```python
from build123d import *

# Parameters (mm, degrees)
SKETCH1_R           = 4
SKETCH1_R_2         = 1.5
SKETCH1_R_3         = 2
BOSS_EXTRUDE1_DEPTH = 2.5
SKETCH2_R           = 2.1
BOSS_EXTRUDE2_DEPTH = 9.5


with BuildPart() as part:
    # Sketch1 → Boss-Extrude1 (new body)
    with BuildSketch(Plane.XY):
        with BuildLine():
            Line((-24, 5.07179677), (-24, 21.07179677))
            Line((-24, 21.07179677), (-4, 33.07179677))
            Line((-4, 33.07179677), (4, 33.07179677))
            Line((4, 33.07179677), (24, 21.07179677))
            Line((24, 21.07179677), (24, 5.07179677))
            Line((24, 5.07179677), (8, -6.92820323))
            Line((8, -6.92820323), (8, -34.92820323))
            ThreePointArc((8, -34.92820323), (7.414213562, -36.342416793), (6, -36.92820323))
            Line((6, -36.92820323), (-6, -36.92820323))
            ThreePointArc((-6, -36.92820323), (-7.414213562, -36.342416793), (-8, -34.92820323))
            Line((-8, -34.92820323), (-8, -6.92820323))
            Line((-8, -6.92820323), (-24, 5.07179677))
        make_face()
        with Locations((-12, 14.07179677)):
            Circle(SKETCH1_R, mode=Mode.SUBTRACT)
        with Locations((-4, 14.07179677)):
            Circle(SKETCH1_R_2, mode=Mode.SUBTRACT)
        with Locations((4, 14.07179677)):
            Circle(SKETCH1_R_2, mode=Mode.SUBTRACT)
        with Locations((0, 29.07179677)):
            Circle(SKETCH1_R_2, mode=Mode.SUBTRACT)
        with Locations((20, 17.07179677)):
            Circle(SKETCH1_R_2, mode=Mode.SUBTRACT)
        with Locations((20, 9.07179677)):
            Circle(SKETCH1_R_2, mode=Mode.SUBTRACT)
        with Locations((-20, 17.07179677)):
            Circle(SKETCH1_R_2, mode=Mode.SUBTRACT)
        with Locations((-20, 9.07179677)):
            Circle(SKETCH1_R_2, mode=Mode.SUBTRACT)
        with Locations((13, 14.07179677)):
            Circle(SKETCH1_R_3, mode=Mode.SUBTRACT)
        with BuildLine():
            Line((4, -30.92820323), (-4, -30.92820323))
            Line((-4, -30.92820323), (-4, -6.92820323))
            ThreePointArc((-4, -6.92820323), (0, 8), (4, -6.92820323))
            Line((4, -6.92820323), (4, -30.92820323))
        make_face(mode=Mode.SUBTRACT)
        with BuildLine():
            Line((-5, 25.07179677), (5, 25.07179677))
            ThreePointArc((5, 25.07179677), (6.414213562, 24.486010332), (7, 23.07179677))
            Line((7, 23.07179677), (7, 20.07179677))
            ThreePointArc((7, 20.07179677), (6.414213562, 18.657583207), (5, 18.07179677))
            Line((5, 18.07179677), (-5, 18.07179677))
            ThreePointArc((-5, 18.07179677), (-6.414213562, 18.657583207), (-7, 20.07179677))
            Line((-7, 20.07179677), (-7, 23.07179677))
            ThreePointArc((-7, 23.07179677), (-6.414213562, 24.486010332), (-5, 25.07179677))
        make_face(mode=Mode.SUBTRACT)
    extrude(amount=BOSS_EXTRUDE1_DEPTH)

    # Sketch2 → Boss-Extrude2 (add)
    with BuildSketch(Plane(origin=(0, 0, 0), x_dir=(-1, 0, 0), z_dir=(0, 0, -1))):
        with Locations(Location((-5, -32.16164975, 0), (0, 0, 61.563109851))):
            Circle(SKETCH2_R)
        with Locations(Location((5, -32.16164975, 0), (0, 0, 144.030430851))):
            Circle(SKETCH2_R)
    extrude(amount=BOSS_EXTRUDE2_DEPTH)


solid = part.part
```
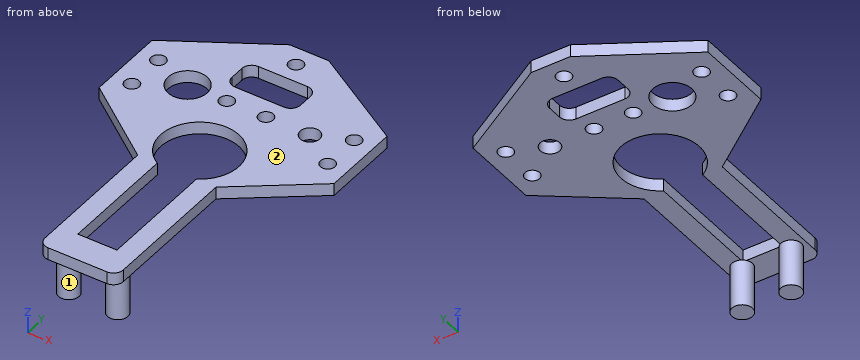
CAD build for the part. Positions are in the model's coordinates, mm. Face numbers are marked on the shaded views. Give positions to 0.01 mm unless a question says otherwise; leave off trailing zeros. Order: outer loops, then holes, each group sorted by start corner. A loop starts at its lowest first (then second) coordinate and runs counter-clockwise, first axis right, second up.
(1) Flat gauge pins, fed straight in: pin 1 (5 mm diameter, centred on x = 0, y = 29.07, fed in from -Z); pin 2 (0.7 mm diameter, centred on x = 3.5, y = -30.5, fed in from +Z); pin 3 (2 mm diameter, centred on y = -20.5, z = 1, fed in from +X); pin 4 (2 mm diameter, centred on x = -13.5, z = -2, fed in from -Y). Where does each tip first touch, or does it go through?
(2) Saw through at A-A, the plane y = -16. Give the cut face in (x, z).
(3) Saw through at B-B, the plane x = 13. Give the cut face in (y, z).
(4) Drill centre lines: L1, parallel to Y at x = 0, z = 0.65; L2, parallel to X at y = -34, z = -5.75; L3, parallel to Y at x = -20, z = 1.9. Where is each one in solid material? Low to high.
(5) Mould opens along X. For the marked faces 1 and 2 say: released by +X, released by -X, zero draft, split by the parting line, or undercut.
(6) Saw through at D-D, the plane z = -1.25. Give the cut face in (x, y).
(7) Saw through at C-C, the plane x = 0. Give the cut face in (y, z), then the cut area to 3 significant figures.
Results found:
1. pin 1: stops at z = 0
1. pin 2: stops at z = 0
1. pin 3: stops at x = 8
1. pin 4: passes through
2. outline: (-8, 0) - (-4, 0) - (-4, 2.5) - (-8, 2.5) - close; (4, 0) - (8, 0) - (8, 2.5) - (4, 2.5) - close
3. outline: (-3.18, 0) - (12.07, 0) - (12.07, 2.5) - (-3.18, 2.5) - close; (16.07, 0) - (27.67, 0) - (27.67, 2.5) - (16.07, 2.5) - close
4. L1: y = -36.93 to -30.93, 8 to 18.07, 25.07 to 27.57, 30.57 to 33.07
4. L2: x = -6.02 to -3.98, 3.98 to 6.02
4. L3: y = 2.07 to 7.57, 10.57 to 15.57, 18.57 to 23.47
5. face 1: undercut
5. face 2: zero draft
6. outline: circle Ø4.2 at (-5, -32.16); circle Ø4.2 at (5, -32.16)
7. outline: (-36.93, 0) - (-30.93, 0) - (-30.93, 2.5) - (-36.93, 2.5) - close; (8, 0) - (18.07, 0) - (18.07, 2.5) - (8, 2.5) - close; (25.07, 0) - (27.57, 0) - (27.57, 2.5) - (25.07, 2.5) - close; (30.57, 0) - (33.07, 0) - (33.07, 2.5) - (30.57, 2.5) - close
7. area: 52.7 mm2
